Here's the drawing with two shaded views (mm, measured from the low corner). I have some questions. A direction names the side the tool comes from. Coordinates: 2 decimals unless noted, no trailing zeros. Write each loop counter-clockwise with the first axis right and the second up, starting at its lowest first coordinate (ties: lowest second). Pieces come first, ordered by that corner, then holes. Notation, with made-up numbers: (-24, 34.5) -> (11, 34.5) arc R15 ccw to (11, 45.5) -> close; hole circle Ø10 at (-12.75, 88.5). An arc over 180 degrees is marked (long way). Answer in a Markdown table with one row per item. Add a question column.
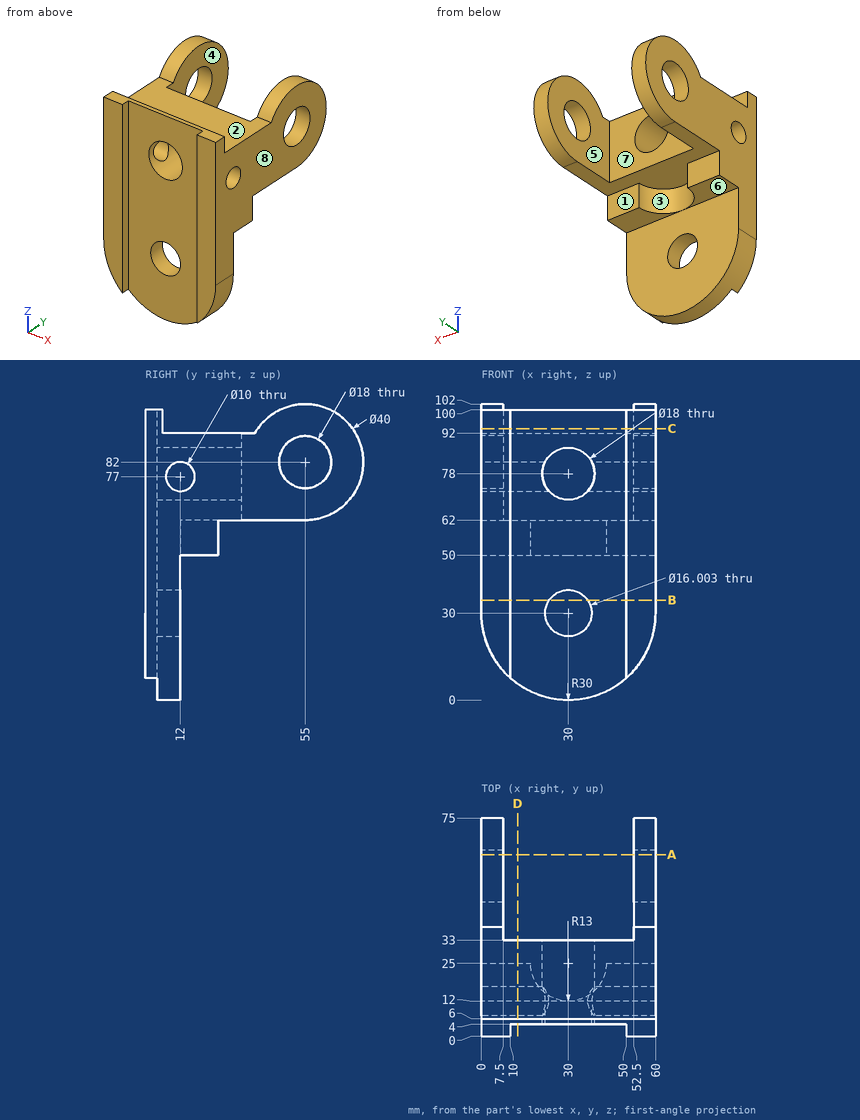
Q1. Imagine slicing it at D-D on x = 12.5. Please give me the cut outline in (y, z).
Q2. I need wall thicknesses on line 1 (X direction, y = 3.5, z = 38.5); line 2 (X direction, y = 6.25, z = 30); line 3 (Z direction, x = 29.5, y = 25.5). Which ranges of each line are inside material? Lowest first, please. Write a range as [from, to].
Q3. For the marked faces 1, 2, 3 and 4, which set-ups out of +Z, -Z, +X, -X, +Y, -Y let a thin tool reach every point of the face, with its end or its side?
Q4. Imagine slicing it at C-C on z = 93.5. Please give me the cut outline in (x, y).
Q5. I'm going to push flat-ended pins straight in: P1, Ø4, axis at x = 19, z = 64, coming from the -Y side; P2, Ø4, axis at x = 50.5, y = 19.5, coming from the -Z side; P3, Ø24, axis at x = 19, z = 78.5, coming from the +Y side. Where does each tip first touch, or does it pass through?
Q6. If we mould it in two halves opening along X, with no side actions, what happens to the marked faces 5, 6, 7 and 8? For each: pulls with the +X half, pulls with the -X half, needs draft (parallel to the pull), parting line crosses it, or undercut.
Q7. Imagine slicing it at A-A on y = 62.5. Please give me the cut outline in (x, z) (1 decimal), plus the area to 3 significant figures.
Q8. Imagine slicing it at B-B on z = 34.5. Please give me the cut outline in (x, y).
Result sheet:
| question | item | result |
|---|---|---|
| 1 | outline | (4, 5.63) -> (12, 5.63) -> (12, 50) -> (25, 50) -> (25, 62) -> (33, 62) -> (33, 92) -> (6, 92) -> (6, 100) -> (4, 100) -> close; hole circle Ø10 at (12, 77) |
| 2 | line 1 | x = [0, 10], [50, 60] |
| 2 | line 2 | x = [0, 22], [38, 60] |
| 2 | line 3 | z = [62, 69.01], [86.99, 92] |
| 3 | face 1 | -Z, +X, -X, +Y |
| 3 | face 2 | +Z, +X, -X |
| 3 | face 3 | -Z, +Y |
| 3 | face 4 | +Z, -Z, +Y |
| 4 | outline | (0, 0) -> (10, 0) -> (10, 4) -> (50, 4) -> (50, 0) -> (60, 0) -> (60, 6) -> (0, 6) -> close; (0, 38.64) -> (7.5, 38.64) -> (7.5, 71.36) -> (0, 71.36) -> close; (52.5, 38.64) -> (60, 38.64) -> (60, 71.36) -> (52.5, 71.36) -> close |
| 5 | P1 | stops at y = 4 |
| 5 | P2 | stops at z = 50 |
| 5 | P3 | stops at y = 75 |
| 6 | face 5 | undercut |
| 6 | face 6 | needs draft |
| 6 | face 7 | undercut |
| 6 | face 8 | pulls with the +X half |
| 7 | outline | (0, 63.5) -> (7.5, 63.5) -> (7.5, 77) -> (0, 77) -> close; (0, 87) -> (7.5, 87) -> (7.5, 100.5) -> (0, 100.5) -> close; (52.5, 63.5) -> (60, 63.5) -> (60, 77) -> (52.5, 77) -> close; (52.5, 87) -> (60, 87) -> (60, 100.5) -> (52.5, 100.5) -> close |
| 7 | area | 407 mm^2 |
| 8 | outline | (0, 0) -> (10, 0) -> (10, 4) -> (23.38, 4) -> (23.38, 12) -> (0, 12) -> close; (36.62, 4) -> (50, 4) -> (50, 0) -> (60, 0) -> (60, 12) -> (36.62, 12) -> close |
